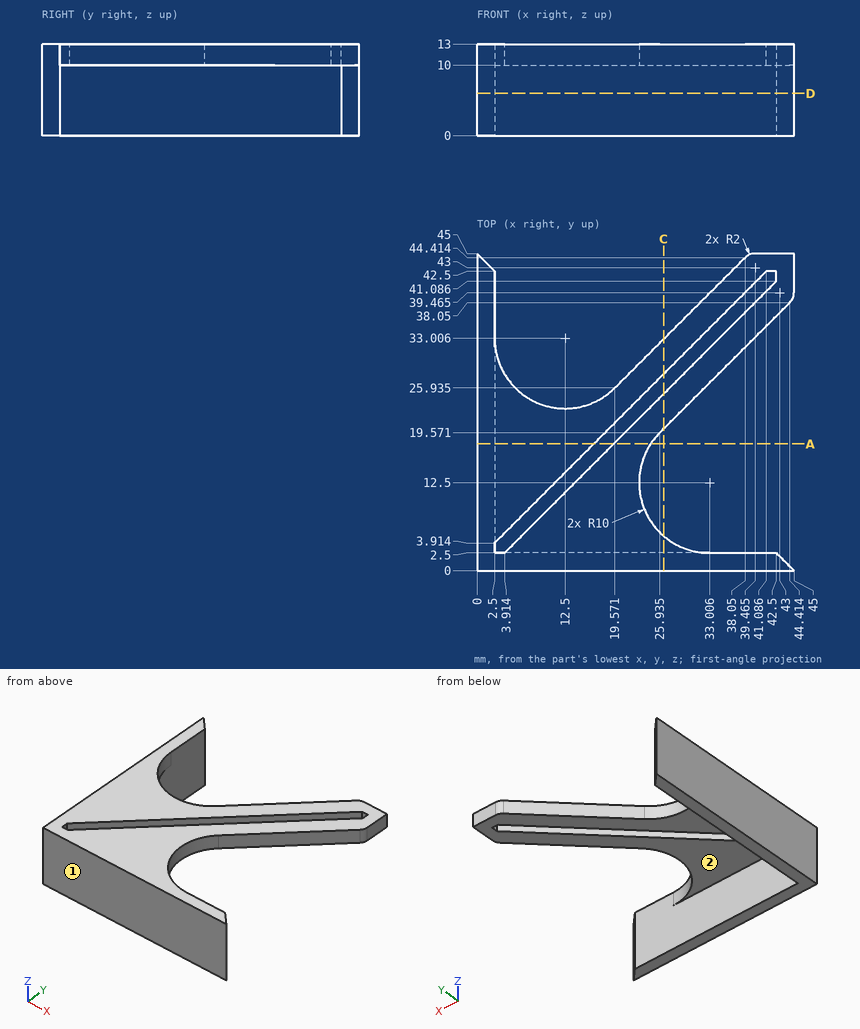
Part print with two shaded views. Sizes in mm from the minimum x, y, z corner. A direction names the side the tool comes from. Round coordinates to 2 decimals unless told otherwise and drop trailing zeros. Write each loop counter-clockwise with the first axis right and the second up, starting at its lowest first coordinate (ties: lowest second). Pieces come first, ordered by that corner, then holes. Notation, with made-up numbers: M 81,84.25 L 134,84.25 A25 cw 134,97.25 Z; hole C 73.25,28 d1. An arc over 180 degrees is marked long. Answer as CSV lines item,"result". Start each with the question number.
1) Which spindle directions (+Z, -Z, +X, -X, +Y, -Y) get a long thin tool onto all of the face, cutting with end or side? Do the marked faces 1 and 2. Say none if no direction does.
2) Drill centre lines: L1, parallel to Y at x = 41.5, z = 12 (1 decimal); L2, parallel to X at y = 36, z = 11 (1 decimal); L3, parallel to Y at x = 39, z = 10.75 (1 decimal). Where is each one in solid material? Low to high.
3) Band-saw the part on D-D (z = 6). List the corners of the cut face in (x, y).
4) Drop flat-ended pins along their axis: pin 1 (13 mm diameter, centred on x = 15.5, y = 19.5, fed in from -Z); pin 2 (2 mm diameter, centred on y = 38, z = 5.5, fed in from +X); pin 3 (1 mm diameter, centred on x = 31.5, z = 6.5, fed in from +Y). Give the stop position or say it passes through.
5) Band-saw the part on C-C (x = 26.5). List the corners of the cut face in (y, z) (1 decimal).
6) Band-saw the part on A-A (y = 18). List the corners of the cut face in (x, z) (1 decimal).
Worked out:
1,face 1,"+Z, -Z, +X, -X, -Y"
1,face 2,"-Z, +X, +Y"
2,L1,"0 to 2.5, 35.1 to 40.1, 42.5 to 45"
2,L2,"0 to 2.5, 29.6 to 34.6, 37.4 to 42.4"
2,L3,"0 to 2.5, 32.6 to 37.6, 40.4 to 44.9"
3,outline,"M 0,0 L 45,0 L 42.5,2.5 L 2.5,2.5 L 2.5,42.5 L 0,45 Z"
4,pin 1,"z = 10"
4,pin 2,"x = 2.5"
4,pin 3,"y = 2.5"
5,outline,"M 0,0 L 2.5,0 L 2.5,10 L 4.9,10 L 4.9,13 L 0,13 Z; M 20.1,10 L 25.1,10 L 25.1,13 L 20.1,13 Z; M 27.9,10 L 32.9,10 L 32.9,13 L 27.9,13 Z"
6,outline,"M 0,0 L 2.5,0 L 2.5,10 L 16.6,10 L 16.6,13 L 0,13 Z; M 19.4,10 L 24.7,10 L 24.7,13 L 19.4,13 Z"
